CAD build for the part. Positions are in the model's coordinates, mm. Face numbers are marked on the shaded views. A direction names the side the tool comes from. Round coordinates to 2 decimals unless told otherwise and drop trailing zeros. Order: outer loops, then holes, each group sorted by start corner. A loop starts at its lowest first (then second) coordinate and runs counter-clockwise, first axis right, second up. Notation, with made-up numbers: (19.25, 31) - (24.25, 31) arc R14 ccw to (24.25, 35) - close; hole circle Ø8 at (63.25, 86.5). An arc over 180 degrees is marked (long way). Write item = value, one per line.
from build123d import *

# Parameters (mm, degrees)
SKETCH1_R                = 11.1125
BOSS_EXTRUDE1_DEPTH      = 38.1
BOSS_EXTRUDE2_DEPTH      = 12.7
BOSS_EXTRUDE2_DEPTH_BACK = 12.7
SKETCH2_W                = 9.525
SKETCH2_H                = 31.75
BOSS_EXTRUDE3_DEPTH      = 12.7
BOSS_EXTRUDE3_DEPTH_BACK = 12.7
SKETCH3_W                = 63.5
SKETCH3_H                = 19.05
BOSS_EXTRUDE4_DEPTH      = 12.7
BOSS_EXTRUDE4_DEPTH_BACK = 12.7
SKETCH4_W                = 19.05
SKETCH4_H                = 69.85
BOSS_EXTRUDE5_DEPTH      = 12.7
BOSS_EXTRUDE5_DEPTH_BACK = 12.7
FILLET1_R                = 6.35


with BuildPart() as part:
    # Sketch1 → Boss-Extrude1 (new body)
    with BuildSketch(Plane(origin=(0, 0, 0), x_dir=(0, 0, -1), z_dir=(1, 0, 0))):
        Circle(SKETCH1_R)
    extrude(amount=-BOSS_EXTRUDE1_DEPTH)

    # Sketch2 → Boss-Extrude2 (add, two sides: drawn at the far end of the back side and taken through both)
    with BuildSketch(Plane.XY.offset(-BOSS_EXTRUDE2_DEPTH_BACK)):
        with Locations((4.7625, 4.7625)):
            Rectangle(SKETCH2_W, SKETCH2_H)
    extrude(amount=BOSS_EXTRUDE2_DEPTH + BOSS_EXTRUDE2_DEPTH_BACK)

    # Sketch3 → Boss-Extrude3 (add, two sides: drawn at the far end of the back side and taken through both)
    with BuildSketch(Plane.XY.offset(-BOSS_EXTRUDE3_DEPTH_BACK)):
        with Locations((-22.225, 30.1625)):
            Rectangle(SKETCH3_W, SKETCH3_H)
    extrude(amount=BOSS_EXTRUDE3_DEPTH + BOSS_EXTRUDE3_DEPTH_BACK)

    # Sketch4 → Boss-Extrude4 (add, two sides: drawn at the far end of the back side and taken through both)
    with BuildSketch(Plane.XY.offset(-BOSS_EXTRUDE4_DEPTH_BACK)):
        with Locations((-44.45, 55.5625)):
            Rectangle(SKETCH4_W, SKETCH4_H)
    extrude(amount=BOSS_EXTRUDE4_DEPTH + BOSS_EXTRUDE4_DEPTH_BACK)

    # Sketch5 → Boss-Extrude5 (add, two sides: drawn at the far end of the back side and taken through both)
    with BuildSketch(Plane.XY.offset(-BOSS_EXTRUDE5_DEPTH_BACK)):
        Polygon((-53.975, 77.7875), (-41.23944, 77.7875), (-41.23944, 80.9625), (-28.575, 80.9625), (-28.575, 90.4875), (-53.975, 90.4875), align=None)
    extrude(amount=BOSS_EXTRUDE5_DEPTH + BOSS_EXTRUDE5_DEPTH_BACK)

    # Fillet1
    fillet1_edges = [part.edges().sort_by_distance(p)[0] for p in [
        (-34.925, 39.6875, 0),
    ]]
    fillet(fillet1_edges, radius=FILLET1_R)


solid = part.part
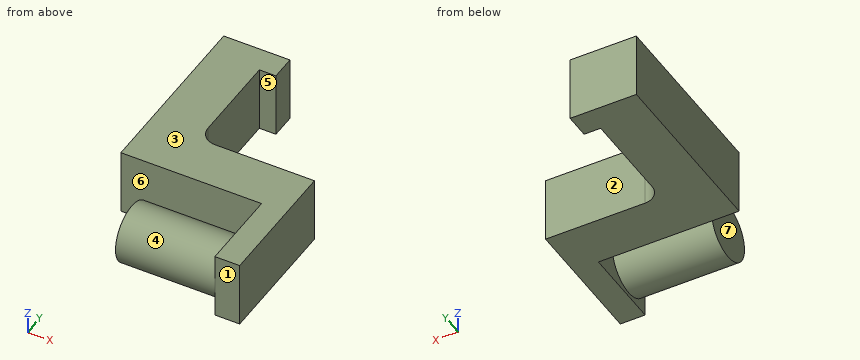
(1) Band-saw the part on D-D on x = -41.5. List the corners of the cut face in (y, z), plus the area to 3 significant figures.
Solved:
outline = (20.64, -12.7) - (90.49, -12.7) - (90.49, 12.7) - (20.64, 12.7) - close
area = 1,770 mm²
(2) Band-saw the part on B-B on y = 0. List the corners of the cut face in (x, z) (1 decimal), plus the area to 3 significant figures.
Solved:
outline = (-38.1, -11.1) - (0, -11.1) - (0, -12.7) - (9.5, -12.7) - (9.5, 12.7) - (0, 12.7) - (0, 11.1) - (-38.1, 11.1) - close
area = 1,090 mm²
(3) Tool access for the marked faces 5, 6 and 7: list every direction of +Z, -Z, +X, -X, +Y, -Y with a clear straight run to the whole face (end or side of a thin tool).
Solved:
face_5 = +Z, -Z, +X
face_6 = +Z, -Z, -X
face_7 = +Z, -Z, -X, -Y
(4) Drop flat-ended pins along their axis: pin 1 (4 mm diameter, centred on x = -14.5, z = -5.5, fed in from +Y); pin 2 (4 mm diameter, centred on x = -12.5, y = 6, fed in from -Z); pin 3 (2 mm diameter, centred on x = -16.5, y = 5.5, fed in from +Z). Give the stop position or say it passes through.
Solved:
pin_1 = 39.69
pin_2 = -10.37
pin_3 = 10.16
(5) Probe line 1 along X through (y, z) = (80.5, -0.75) (3 decimals); line 2 along X through (y, z) = (82.5, -1.25) (3 decimals); line 3 along Y through (x, z) = (-20, -1.25). List the from-to ranges inside material, lowest first.
Solved:
line_1 = -53.975 to -34.925
line_2 = -53.975 to -28.575
line_3 = -11.04 to 11.04, 20.64 to 39.69
(6) Pull direction Y, two halves, no side cores. Call the marked faces 1, 2, 3 and 4: released by +Y, released by -Y, zero draft, split by the parting line, or undercut.
Solved:
face_1 = released by -Y
face_2 = released by +Y
face_3 = zero draft
face_4 = undercut
(7) Band-saw the part on A-A on x = -4. List the corners of the cut face in (y, z) (1 decimal).
Solved:
outline = circle Ø22.2 at (0, 0); (20.6, -12.7) - (39.7, -12.7) - (39.7, 12.7) - (20.6, 12.7) - close
